CAD build for the part. Positions are in the model's coordinates, mm. A direction names the side the tool comes from. Give positions to 0.01 mm unless a question says otherwise; leave off trailing zeros. Order: outer loops, then holes, each group sorted by start corner. A loop starts at its lowest first (then second) coordinate and runs counter-clockwise, first axis right, second up.
from build123d import *

# Parameters (mm, degrees)
ESQUISSE1_W             = 22.5
ESQUISSE1_H             = 10
BOSS_EXTRU_1_DEPTH      = 8
CHANFREIN1_SIZE         = 2
BOSS_EXTRU_3_DEPTH      = 6.5
ENL_V_MAT_EXTRU_1_DEPTH = 7
TROU_TARAUD_M33_D       = 2.5
CONG_1_R                = 0.5


with BuildPart() as part:
    # Esquisse1 → Boss.-Extru.1 (new body)
    with BuildSketch(Plane.XY):
        with Locations((11.25, 5)):
            Rectangle(ESQUISSE1_W, ESQUISSE1_H)
    extrude(amount=BOSS_EXTRU_1_DEPTH)

    # Chanfrein1
    chanfrein1_edges = [part.edges().sort_by_distance(p)[0] for p in [
        (0, 5, 0),
    ]]
    chamfer(chanfrein1_edges, length=CHANFREIN1_SIZE)

    # Esquisse3 → Boss.-Extru.3 (add)
    with BuildSketch(Plane.ZY):
        Polygon((8, 10), (21.413248654, 10), (24.3, 5), (21.413248654, 0), (8, 0), (2, 0), (2, 10), align=None)
    extrude(amount=-BOSS_EXTRU_3_DEPTH)

    # Esquisse4 → Enlèv. mat.-Extru.1 (cut)
    with BuildSketch(Plane(origin=(0, 10, 0), x_dir=(1, 0, 0), z_dir=(0, 1, 0))):
        with BuildLine():
            Line((0, -8.5), (2, -8.5))
            ThreePointArc((2, -8.5), (4, -10.5), (2, -12.5))
            Line((2, -12.5), (0, -12.5))
            Line((0, -12.5), (0, -8.5))
        make_face()
    extrude(amount=-ENL_V_MAT_EXTRU_1_DEPTH, mode=Mode.SUBTRACT)

    # Trou taraudé M33 (through all)
    with Locations(Plane(origin=(19.5, 5, 0), x_dir=(-1, 0, 0), z_dir=(0, 0, -1))):
        with Locations((0, 0), (7, 0)):
            Hole(TROU_TARAUD_M33_D / 2)

    # Congé1
    cong_1_edges = [part.edges().sort_by_distance(p)[0] for p in [
        (0, 10, 5.25),
        (3.25, 5, 24.3),
        (3.25, 0, 21.413248654),
        (14.5, 0, 8),
        (12.25, 0, 0),
        (1, 0, 1),
        (2, 5, 0),
        (1, 3, 8.5),
        (4, 3, 10.5),
        (1, 3, 12.5),
        (22.5, 0, 4),
        (22.5, 5, 8),
        (22.5, 5, 0),
        (6.5, 2.5, 22.856624327),
        (6.5, 7.5, 22.856624327),
        (6.5, 5, 8),
        (6.5, 0, 14.706624327),
        (1, 10, 1),
        (12.25, 10, 0),
        (22.5, 10, 4),
        (14.5, 10, 8),
        (6.5, 10, 14.706624327),
        (3.25, 10, 21.413248654),
        (1, 10, 12.5),
        (4, 10, 10.5),
        (1, 10, 8.5),
        (0, 6.5, 12.5),
        (0, 10, 16.956624327),
        (0, 7.5, 22.856624327),
        (0, 2.5, 22.856624327),
        (0, 0, 11.706624327),
        (0, 5, 2),
        (0, 6.5, 8.5),
        (0, 3, 10.5),
    ]]
    fillet(cong_1_edges, radius=CONG_1_R)


solid = part.part
1. Saw through at A-A on x = 19.5. Give the cut face in (y, z), plus the area to 3 significant figures.
2. Saw through at D-D on x = 8.25. Give the cut face in (y, z), plus the area to 3 significant figures.
3. Saw through at B-B on z = 18.75. Give the cut face in (x, y).
4. Saw through at C-C on z = 5.75. Give the cut face in (x, y).
5. Wall check: line 1 (Y direction, x = 12.5, z = 5.75); line 2 (Z direction, x = 20.75, y = 8.25); line 3 (X direction, y = 1, z = 20). Give the ranges that are in metal, low to high.
6. 3-axis set-ups, long thin cutter, end or side, ignore diameter. For faces 4 (the flat face through (14, 5, 8)), 5 (the flat face through (2, 3, 10)), 6 (the flat face through (9, 0, 6)): which of +Z, -Z, +X, -X, +Y, -Y reach the whole face in a straight line?
7. Pin check, flat tips, straight feed: P1, Ø0.8, axis at x = 1, y = 8, coming from the -Z side; P2, Ø2.5, axis at x = 2, z = 11, coming from the +Y side; P3, Ø4, axis at x = 12.5, y = 5, coming from the +Z side. Stop position of each tip, or through.
8. Mould opens along Z. For faces 1 (the flat face through (1, 7, 12.5)), 2 (the flat face through (12, 3, 0)), 3 (the cylindrical face through (20.655, 4.521, 4.056)) say: released by +Z, released by -Z, zero draft, split by the parting line, or undercut.
Reported:
1. outline: (0, 0.5) arc R0.5 ccw to (0.5, 0) - (3.75, 0) - (3.75, 8) - (0.5, 8) arc R0.5 ccw to (0, 7.5) - close; (6.25, 0) - (9.5, 0) arc R0.5 ccw to (10, 0.5) - (10, 7.5) arc R0.5 ccw to (9.5, 8) - (6.25, 8) - close
1. area: 59.8 mm2
2. outline: (0, 0.5) arc R0.5 ccw to (0.5, 0) - (9.5, 0) arc R0.5 ccw to (10, 0.5) - (10, 7.5) arc R0.5 ccw to (9.5, 8) - (0.5, 8) arc R0.5 ccw to (0, 7.5) - close
2. area: 79.8 mm2
3. outline: (0, 0.5) arc R0.5 ccw to (0.5, 0) - (6, 0) arc R0.5 ccw to (6.5, 0.5) - (6.5, 9.5) arc R0.5 ccw to (6, 10) - (0.5, 10) arc R0.5 ccw to (0, 9.5) - close
4. outline: (0, 0.5) arc R0.5 ccw to (0.5, 0) - (22, 0) arc R0.5 ccw to (22.5, 0.5) - (22.5, 9.5) arc R0.5 ccw to (22, 10) - (0.5, 10) arc R0.5 ccw to (0, 9.5) - close; hole circle Ø2.5 at (12.5, 5); hole circle Ø2.5 at (19.5, 5)
5. line 1: y = 0 to 3.75, 6.25 to 10
5. line 2: z = 0 to 8
5. line 3: x = 0 to 6.5
6. face 4: +Z, +X, +Y, -Y
6. face 5: -X, +Y
6. face 6: +Z, -Z, +X, -X, -Y
7. P1: stops at z = 0.6
7. P2: stops at y = 3.07
7. P3: stops at z = 8
8. face 1: undercut
8. face 2: released by -Z
8. face 3: zero draft
